Read the model definition and answer for the solid it produces. Units are mm, in the model's axes. A direction names the side the tool comes from. Coordinates: 2 decimals unless noted, no trailing zeros. Order: outer loops, then holes, each group sorted by start corner. A loop starts at its lowest first (then second) coordinate and runs counter-clockwise, first axis right, second up. Notation, with made-up numbers: (-22.5, 56) - (0.5, 56) arc R33 ccw to (0.5, 92) - close; hole circle Ø7 at (2, 15.5). An arc over 180 degrees is marked (long way). Write item = value, one per line.
from build123d import *

# Parameters (mm, degrees)
SKETCH1_W           = 57.15
SKETCH1_H           = 101.6
BOSS_EXTRUDE1_DEPTH = 3.175
SKETCH2_W           = 57.15
SKETCH2_H           = 57.15
BOSS_EXTRUDE2_DEPTH = 6.35
SKETCH4_R           = 3
CUT_EXTRUDE2_DEPTH  = 7.35
CUT_EXTRUDE3_DEPTH  = 7.35
FILLET1_R           = 6.35


with BuildPart() as part:
    # Sketch1 → Boss-Extrude1 (new body, symmetric)
    with BuildSketch(Plane.XY):
        Rectangle(SKETCH1_W, SKETCH1_H)
    extrude(amount=BOSS_EXTRUDE1_DEPTH, both=True)

    # Sketch2 → Boss-Extrude2 (add)
    with BuildSketch(Plane.XZ.offset(50.8)):
        with Locations((0, 25.4)):
            Rectangle(SKETCH2_W, SKETCH2_H)
    extrude(amount=-BOSS_EXTRUDE2_DEPTH)

    # Sketch4 → Cut-Extrude2 (cut, through all)
    with BuildSketch(Plane(origin=(0, -44.45, 0), x_dir=(1, 0, 0), z_dir=(0, 1, 0))):
        with Locations((0, -28.575)):
            Circle(SKETCH4_R)
    extrude(amount=-CUT_EXTRUDE2_DEPTH, mode=Mode.SUBTRACT)

    # Sketch5 → Cut-Extrude3 (cut, through all)
    with BuildSketch(Plane(origin=(0, -44.45, 0), x_dir=(1, 0, 0), z_dir=(0, 1, 0))):
        Polygon((-28.575, -3.175), (-6.35, -34.925), (6.35, -34.925), (28.575, -3.175), (28.575, -53.975), (-28.575, -53.975), align=None)
    extrude(amount=-CUT_EXTRUDE3_DEPTH, mode=Mode.SUBTRACT)

    # Fillet1
    fillet1_edges = [part.edges().sort_by_distance(p)[0] for p in [
        (-6.35, -47.625, 34.925),
        (6.35, -47.625, 34.925),
    ]]
    fillet(fillet1_edges, radius=FILLET1_R)


solid = part.part
1) Flat-ended cylindrical pins translate along their axes: pin 1 Ø1.5 at (x, y) = (-22.5, -26.5) entering from +Z (3 decimals); pin 2 Ø16 at (x, z) = (-8.5, 19.5) entering from +Y. Find the tip coordinate at first contact, or state that the pin passes through.
Returned:
pin_1 = 3.175
pin_2 = -44.45
2) Determine the mould class of faces 1 (the face through (5.938, -47.669, 34.227)), 2 (the face through (0, -50.8, 12)), 3 (the face through (-0.65, -47.581, 31.504)) for opening direction Z: pulls with the +Z half, pulls with the -Z half, needs draft (parallel to the pull), parting line crosses it, or undercut.
Returned:
face_1 = pulls with the +Z half
face_2 = needs draft
face_3 = undercut
3) The part is cut by section D-D (x = -6). Determine the outline of the cut face in (y, z) (3 decimals), and give its area (3 significant figures).
Returned:
outline = (-50.8, -3.175) - (50.8, -3.175) - (50.8, 3.175) - (-44.45, 3.175) - (-44.45, 34.195) - (-50.8, 34.195) - close
area = 842 mm^2
4) The part is cut by section A-A (x = 0). Determine the outline of the cut face in (y, z) (3 decimals).
Returned:
outline = (-50.8, -3.175) - (50.8, -3.175) - (50.8, 3.175) - (-44.45, 3.175) - (-44.45, 25.575) - (-50.8, 25.575) - close; (-50.8, 31.575) - (-44.45, 31.575) - (-44.45, 34.925) - (-50.8, 34.925) - close
5) The part is cut by section C-C (z = 24.5). Determine the outline of the cut face in (x, y), and give its area (3 significant figures).
Returned:
outline = (-13.65, -50.8) - (13.65, -50.8) - (13.65, -44.45) - (-13.65, -44.45) - close
area = 173 mm^2
6) Straight lines are drawn through the part: line 1 along Z through (x, y) = (0, -49) (3 decimals); line 2 along Z through (x, y) = (-11, 36.5) (3 decimals); line 3 along Y through (x, z) = (-12, 15). For each, find the intervals that lie inside material, in ascending order. Write a range as from..to.
Returned:
line_1 = -3.175..25.575, 31.575..34.925
line_2 = -3.175..3.175
line_3 = -50.8..-44.45
7) The part is cut by section B-B (y = 30). Determine the outline of the cut face in (x, z) (3 decimals), and give its area (3 significant figures).
Returned:
outline = (-28.575, -3.175) - (28.575, -3.175) - (28.575, 3.175) - (-28.575, 3.175) - close
area = 363 mm^2
8) For faces 4 (the face through (28.575, -1, 0)), 5 (the face through (0, -44.45, 16)), determine the directions among +Z, -Z, +X, -X, +Y, -Y from which every point of the face is accessible in a straight line to the end or side of a thin tool.
Returned:
face_4 = +Z, -Z, +X, +Y, -Y
face_5 = +Z, +X, -X, +Y
